Check sheet for the modelled part. Datum: model origin and axes. Units: mm. A direction names the side the tool comes from. Round coordinates to 2 decimals unless told otherwise and drop trailing zeros. Order: outer loops, then holes, each group sorted by start corner. A loop starts at its lowest first (then second) coordinate and runs counter-clockwise, first axis right, second up.
```python
from build123d import *

# Parameters (mm, degrees)
F0_R      = 1.15
F1_DEPTH  = 0.88
F2_DEPTH  = 0.88
F3_W      = 2.8
F3_H      = 3.5
F4_DEPTH  = 2.79
F5_W      = 2.8
F5_H      = 3.5
F6_DEPTH  = 2.79
F8_DEPTH  = 2.79
F10_DEPTH = 2.79


with BuildPart() as f1:
    # F0 (on Top) → F1 (new body)
    with BuildSketch(Plane.XY):
        Polygon((5.85, 40), (-5.85, 40), (-5.85, 0), (-5.85, -40), (-0.88, -40), (-0.88, -15), (0.88, -15), (0.88, -40), (5.85, -40), (5.85, 0), align=None)
        with Locations((-3.365, -36.25)):
            Circle(F0_R, mode=Mode.SUBTRACT)
        with Locations((3.365, -36.25)):
            Circle(F0_R, mode=Mode.SUBTRACT)
        with Locations((-2.925, 25.2)):
            Circle(F0_R, mode=Mode.SUBTRACT)
        with Locations((2.925, 25.2)):
            Circle(F0_R, mode=Mode.SUBTRACT)
    extrude(amount=F1_DEPTH)

    # F0 (on Top) → F2 (join)
    with BuildSketch(Plane.XY):
        Polygon((5.85, 40), (-5.85, 40), (-5.85, 0), (-5.85, -40), (-0.88, -40), (-0.88, -15), (0.88, -15), (0.88, -40), (5.85, -40), (5.85, 0), align=None)
        with Locations((-3.365, -36.25)):
            Circle(F0_R, mode=Mode.SUBTRACT)
        with Locations((3.365, -36.25)):
            Circle(F0_R, mode=Mode.SUBTRACT)
        with Locations((-2.925, 25.2)):
            Circle(F0_R, mode=Mode.SUBTRACT)
        with Locations((2.925, 25.2)):
            Circle(F0_R, mode=Mode.SUBTRACT)
    extrude(amount=-F2_DEPTH)

    # F3 (on Top) → F4 (join)
    with BuildSketch(Plane.XY):
        with Locations((3.365, -30.75)):
            Rectangle(F3_W, F3_H)
    extrude(amount=F4_DEPTH)

    # F5 (on Top) → F6 (join)
    with BuildSketch(Plane.XY):
        with Locations((-3.365, -30.75)):
            Rectangle(F5_W, F5_H)
    extrude(amount=-F6_DEPTH)

    # F7 (on Top) → F8 (join)
    with BuildSketch(Plane.XY):
        Polygon((-1.965, -1.75), (-1.965, 0), (-1.965, 1.75), (-4.765, 1.75), (-4.765, 0), (-4.765, -1.75), align=None)
    extrude(amount=F8_DEPTH)

    # F9 (on Top) → F10 (join)
    with BuildSketch(Plane.XY):
        Polygon((1.965, -1.75), (4.765, -1.75), (4.765, 0), (4.765, 1.75), (1.965, 1.75), (1.965, 0), align=None)
    extrude(amount=-F10_DEPTH)


solid = f1.part
```
Item 1: Release check for a two-part mould opening along X. For faces 1 (the flat face through (0.88, -27, 0)), 2 (the flat face through (1.965, -31, 2)), 3 (the flat face through (-0.88, -28, 0)), 4 (the flat face through (3, -40, 0)) record: released by +X, released by -X, zero draft, split by the parting line, or undercut.
Answer:
face 1: undercut
face 2: released by -X
face 3: undercut
face 4: zero draft
Item 2: Access from +Z, -Z, +X, -X, +Y, -Y to the whole of each face (thin tool, end or side, straight path). Record for faces 5 (the flat face through (3, -1.75, -2)), 6 (the flat face through (3, 1.75, -2)), 7 (the flat face through (1.965, 0, -2)), 8 (the flat face through (-1.965, -31, -2)).
Answer:
face 5: -Z, +X, -X, -Y
face 6: -Z, +X, -X, +Y
face 7: -Z, -X, +Y, -Y
face 8: -Z, +X, +Y, -Y
Item 3: Sectioned sample at B-B (y = 25.2). Record the cut outline in (x, z) (3 decimals), and give its area (3 significant figures).
Answer:
outline: (-5.85, -0.88) - (-4.075, -0.88) - (-4.075, 0.88) - (-5.85, 0.88) - close; (-1.775, -0.88) - (1.775, -0.88) - (1.775, 0.88) - (-1.775, 0.88) - close; (4.075, -0.88) - (5.85, -0.88) - (5.85, 0.88) - (4.075, 0.88) - close
area: 12.5 mm2
Item 4: Sectioned sample at A-A (z = 1.8). Record the cut outline in (x, y) (3 decimals), and give its area (3 significant figures).
Answer:
outline: (-4.765, -1.75) - (-1.965, -1.75) - (-1.965, 1.75) - (-4.765, 1.75) - close; (1.965, -32.5) - (4.765, -32.5) - (4.765, -29) - (1.965, -29) - close
area: 19.6 mm2
Item 5: Sectioned sample at D-D (y = -36.25). Record the cut outline in (x, z) (3 decimals).
Answer:
outline: (-5.85, -0.88) - (-4.515, -0.88) - (-4.515, 0.88) - (-5.85, 0.88) - close; (-2.215, -0.88) - (-0.88, -0.88) - (-0.88, 0.88) - (-2.215, 0.88) - close; (0.88, -0.88) - (2.215, -0.88) - (2.215, 0.88) - (0.88, 0.88) - close; (4.515, -0.88) - (5.85, -0.88) - (5.85, 0.88) - (4.515, 0.88) - close
Item 6: Go/stop test with flat-tipped pins: P1, Ø2, axis at x = -3, z = 2, coming from the -Y side; P2, Ø1, axis at y = -30.5, z = -2, coming from the +X side (3 decimals); P3, Ø5, axis at x = 2.5, y = 15, coming from the +Z side. Record where each tip stops, or that it passes through.
Answer:
P1: stops at y = -1.75
P2: stops at x = -1.965
P3: stops at z = 0.88
Item 7: Sectioned sample at C-C (y = -20). Record the cut outline in (x, z).
Answer:
outline: (-5.85, -0.88) - (-0.88, -0.88) - (-0.88, 0.88) - (-5.85, 0.88) - close; (0.88, -0.88) - (5.85, -0.88) - (5.85, 0.88) - (0.88, 0.88) - close
Item 8: Scan lines: line 1 along Z through (x, y) = (-5, 29); line 2 along Y through (x, z) = (3.5, -2); line 3 along Y through (x, z) = (-3, -2.5). Record each from-to range of solid material in increasing order.
Answer:
line 1: z = -0.88 to 0.88
line 2: y = -1.75 to 1.75
line 3: y = -32.5 to -29
